Autodesk Inventor part; units mm, degrees
ref_plane "Work Plane1" through (0, 7, 0) normal (0, 1, 0) x (-1, 0, 0)
ref_plane "YZ Plane" through (0, 0, 0) normal (1, 0, 0) x (0, 1, 0)
ref_plane "XY Plane" through (0, 0, 0) normal (0, 0, 1) x (1, 0, 0)
sketch "Sketch1" plane through (0, 0, 0) normal (0, 0, 1) x (1, 0, 0)
  circle A0 centre (0, 0) radius 5
  circle A1 centre (0, 0) radius 7
  line L0 (-18, -9.5) -> (-10, -9.5)
  line L1 (18, -9.5) -> (10, -9.5)
  line L2 (0, -14) -> (18, -14)
  line L3 (0, -14) -> (-18, -14)
  line L4 (-7, 0) -> (-7, -9.5)
  line L5 (-7, -9.5) -> (-18, -9.5)
  line L6 (-18, -9.5) -> (-18, -14)
  line L7 (-18, -14) -> (18, -14)
  line L8 (18, -14) -> (18, -9.5)
  line L9 (18, -9.5) -> (7, -9.5)
  line L10 (7, -9.5) -> (7, 0)
  point P0 (-10.8595, -8.0551)
  dimension "d0" = 14
  dimension "d1" = 10
  dimension "d2" = 4.5
  dimension "d3" = 0
  dimension "d4" = 11
  dimension "d5" = 36
  dimension "d6" = 9.5
  dimension "d7" = 8
  dimension "d8" = 18
  dimension "d9" = 28
  dimension "d10" = 1.4449
  dimension "d11" = 28.8595
extrude "Extrusion1" add sketch "Sketch1" along normal blind 10
fillet "Fillet1" radius 1 2 edges at (18, -9.5, 5) (-18, -9.5, 5)
fillet "Fillet2" radius 3 2 edges at (7, -9.5, 5) (-7, -9.5, 5)
chamfer "Chamfer1" distance 1 angle 45 22 edges at (0, 7, 10) (-7, -3.2502, 10) (-9.9998, -9.5, 10) (-13.5, -9.5, 10) (-17.7071, -9.7929, 10) (-18, -12.25, 10) (7, -3.2503, 10) (9.9997, -9.5, 10) (13.5, -9.5, 10) (17.7071, -9.7929, 10) (18, -12.25, 10) (0, 7, 0) (-7, -3.2502, 0) (-9.9998, -9.5, 0) (-13.5, -9.5, 0) (-17.7071, -9.7929, 0) (-18, -12.25, 0) (7, -3.2503, 0) (9.9997, -9.5, 0) (13.5, -9.5, 0) (17.7071, -9.7929, 0) (18, -12.25, 0)
sketch "Sketch2" plane through (10, -9.5, 1) normal (0, 1, 0) x (1, 0, 0)
  line L0 (-27, 0) -> (-20, 0)
  line L1 (-27, -8) -> (-27, 0)
  line L2 (-20, -8) -> (-27, -8)
  line L3 (-20, 0) -> (-20, -8)
  line L4 (0, 0) -> (7, 0)
  line L5 (0, -8) -> (0, 0)
  line L6 (7, -8) -> (0, -8)
  line L7 (7, 0) -> (7, -8)
  line L8 (-27, -8) -> (-20, -8)
  line L9 (-20, -8) -> (-20, 0)
  line L10 (-20, 0) -> (-27, 0)
  line L11 (-27, 0) -> (-27, -8)
  line L12 (-27, -8) -> (-20, 0) construction
  line L13 (-20, -8) -> (-27, 0) construction
  line L14 (0, -8) -> (7, -8)
  line L15 (7, -8) -> (7, 0)
  line L16 (7, 0) -> (0, 0)
  line L17 (0, 0) -> (0, -8)
  line L18 (0, -8) -> (7, 0) construction
  line L19 (7, -8) -> (0, 0) construction
  point P0 (-10, 1)
  point P1 (-23.5, -4)
  point P2 (3.5, -4)
  point P3 (-23.5, -4)
  point P4 (3.5, -4)
hole "Hole1" at (-13.5, -9.5, 5) at (13.5, -9.5, 5) direction (0, -1, 0) diameter 2 end through all
ref_plane "Work Plane1" through (0, 7, 0) normal (0, 1, 0) x (-1, 0, 0)
sketch "Sketch3" plane through (0, 7, 0) normal (0, 1, 0) x (-1, 0, 0)
  line L0 (7, 1) -> (-7, 1)
  line L1 (7, 1) -> (7, 9)
  line L2 (-7, 9) -> (7, 9)
  line L3 (-7, 1) -> (-7, 9)
  line L4 (7, 9) -> (-7, 9)
  line L5 (-7, 9) -> (-7, 1)
  line L6 (-7, 1) -> (7, 1)
  line L7 (7, 1) -> (7, 9)
  line L8 (7, 9) -> (-7, 1) construction
  line L9 (-7, 9) -> (7, 1) construction
  point P0 (0, 0)
  point P1 (0, 5)
  point P2 (0, 5)
hole "Hole2" at (0, 7, 5) direction (0, -1, 0) diameter 2 depth 8 tip angle 118 countersink diameter 4 countersink angle 90
properties part number "pt2"
The listing builds one solid part. Answer for the finished solid, in the listing's coordinates (mm). A direction names the side the tool comes from. Coordinates: 2 decimals unless noted, no trailing zeros. Write each loop counter-clockwise with the first axis right and the second up, starting at its lowest first coordinate (ties: lowest second). Pieces come first, ordered by that corner, then holes. Notation, with made-up numbers: (18.5, 2) - (56.5, 2) arc R29 cw to (56.5, 29) - close; hole circle Ø1 at (-27.5, 75). An arc over 180 degrees is marked (long way). Return JSON: item names as keys, results as strings. Group by question number.
Q1. The part is cut by section D-D on z = 5. Write down the section's boundary in (x, y).
Q2. Flat-ended cylindrical pins translate along their axes: pin 1 Ø2 at (x, z) = (12.5, 4) entering from +Y; pin 2 Ø6 at (x, y) = (0, 0) entering from -Z; pin 3 Ø3 at (x, y) = (6, -4) entering from -Z; pin 4 Ø5 at (y, z) = (-2, 4) entering from -X. Find the tip coordinate at first contact, or state that the pin passes through.
Q3. Find the intervals of material crossed by line 1 along X through (y, z) = (-12.2, 5); line 2 along Y through (x, z) = (0, 8); line 3 along Z through (x, y) = (-13.5, -12.35), in increasing order. Write a range as [from, to].
Q4. The part is cut by section A-A on x = 13.5. Write down the section's boundary in (y, z), and give its area (3 significant figures).
Q5. The part is cut by section B-B on z = 2.5. Write down the section's boundary in (x, y).
Q6. The part is cut by section C-C on y = -3.5. Write down the section's boundary in (x, z).
Q7. Which of the six approach directions +Z, -Z, +X, -X, +Y, -Y give full straight-line access (tool end or side, diameter ignored) to faces 1 (the flat face through (6.5, -3.2, 9.5)), 2 (the flat face through (-7, -3, 5)), 3 (the flat face through (-13.5, -10, 0.5)), 4 (the flat face through (-6.5, -3.3, 9.5))?
Evaluation:
{
 "1": {"outline": "(-18, -14) - (-14.5, -14) - (-14.5, -9.5) - (-17, -9.5) arc R1 ccw to (-18, -10.5) - close; (-12.5, -14) - (12.5, -14) - (12.5, -9.5) - (10, -9.5) arc R3 cw to (7, -6.5) - (7, 0) arc R7 ccw to (1.77, 6.77) - (1, 6) - (1, 4.9) arc R5 cw (long way) to (-1, 4.9) - (-1, 6) - (-1.77, 6.77) arc R7 ccw to (-7, 0) - (-7, -6.5) arc R3 cw to (-10, -9.5) - (-12.5, -9.5) - close; (14.5, -14) - (18, -14) - (18, -10.5) arc R1 ccw to (17, -9.5) - (14.5, -9.5) - close"},
 "2": {"pin 1": "stops at y = -9.5", "pin 2": "passes through", "pin 3": "stops at z = 0", "pin 4": "stops at x = -7"},
 "3": {"line 1": "x = [-18, -14.5], [-12.5, 12.5], [14.5, 18]", "line 2": "y = [-14, -5], [5, 7]", "line 3": "z = [0, 4], [6, 10]"},
 "4": {"outline": "(-14, 0) - (-10.5, 0) - (-9.5, 1) - (-9.5, 4) - (-14, 4) - close; (-14, 6) - (-9.5, 6) - (-9.5, 9) - (-10.5, 10) - (-14, 10) - close", "area": "35.0 mm2"},
 "5": {"outline": "(-18, -14) - (18, -14) - (18, -10.5) arc R1 ccw to (17, -9.5) - (10, -9.5) arc R3 cw to (7, -6.5) - (7, 0) arc R7 ccw to (-7, 0) - (-7, -6.5) arc R3 cw to (-10, -9.5) - (-17, -9.5) arc R1 ccw to (-18, -10.5) - close; hole circle Ø10 at (0, 0)"},
 "6": {"outline": "(-7, 1) - (-6, 0) - (-3.57, 0) - (-3.57, 10) - (-6, 10) - (-7, 9) - close; (3.57, 0) - (6, 0) - (7, 1) - (7, 9) - (6, 10) - (3.57, 10) - close"},
 "7": {"face 1": "+Z, +X, +Y", "face 2": "+Z, -Z, -X, +Y", "face 3": "-Z, -X, +Y", "face 4": "+Z, -X, +Y"}
}
